Can you work these out from the model? Positions are in its coordinate system, mm. Face numbers are marked on the shaded views. A direction names the side the tool comes from. Round coordinates to 2 decimals unless told otherwise and drop trailing zeros. Order: outer loops, then holes, each group sorted by start corner. A loop starts at its lowest first (then second) coordinate and runs counter-clockwise, first axis right, second up.
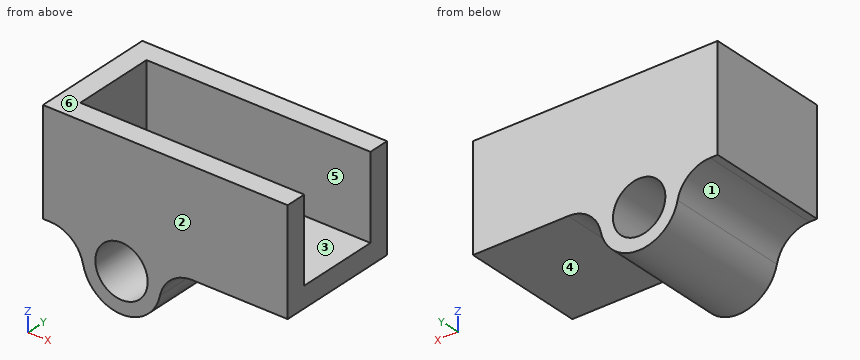
from build123d import *

# Parameters (mm, degrees)
SKETCH1_R           = 2
BOSS_EXTRUDE1_DEPTH = 9.525
FILLET1_R           = 2.54
BOSS_EXTRUDE2_DEPTH = 6.35


with BuildPart() as part:
    # Sketch1 → Boss-Extrude1 (new body)
    with BuildSketch(Plane(origin=(0, 0, 0), x_dir=(1, 0, 0), z_dir=(0, 1, 0))):
        with BuildLine():
            Line((-6, -1.4125), (-6, -3))
            Line((-6, -3), (12.7, -3))
            Line((12.7, -3), (12.7, -1.4125))
            Line((12.7, -1.4125), (2.646666535, -1.4125))
            ThreePointArc((2.646666535, -1.4125), (0, 3), (-2.646666535, -1.4125))
            Line((-2.646666535, -1.4125), (-6, -1.4125))
        make_face()
        Circle(SKETCH1_R, mode=Mode.SUBTRACT)
    extrude(amount=BOSS_EXTRUDE1_DEPTH)

    # Fillet1
    fillet1_edges = [part.edges().sort_by_distance(p)[0] for p in [
        (-2.646666535, 4.7625, 1.4125),
        (2.646666535, 4.7625, 1.4125),
    ]]
    fillet(fillet1_edges, radius=FILLET1_R)

    # Sketch2 → Boss-Extrude2 (add)
    with BuildSketch(Plane.XY.offset(3)):
        Polygon((12.7, 0), (-6, 0), (-6, 9.525), (12.7, 9.525), (12.7, 7.9375), (-4.4125, 7.9375), (-4.4125, 1.5875), (12.7, 1.5875), align=None)
    extrude(amount=BOSS_EXTRUDE2_DEPTH)


solid = part.part
(1) On a 3-axis mill with a long thin cutter (end or side, diameter ignored), from which of +Z, -Z, +X, -X, +Y, -Y can I reach the whole of each face in a straight line? I mean the marked faces 4, 5 and 6. Say none if no direction works.
(2) Please list where these lines run through material, in increasing order: probe 1 along Y at (x, z) = (1.5, 7.75) (1 decimal); probe 2 along X at (y, z) = (6, 7); probe 3 along X at (y, z) = (4.75, 0).
(3) I want a section at B-B, the plane z = 0. List the corners of the cut face in (x, y) for me (3 decimals).
(4) If we mould it in two halves opening along Y, with no side actions, what happens to the marked faces 1, 2 and 3? For each: pulls with the +Y half, pulls with the -Y half, needs draft (parallel to the pull), parting line crosses it, or undercut.
(5) I'm going to push flat-ended pins straight in: pin 1 Ø2 at (x, y) = (7.5, 6.5) entering from -Z; pin 2 Ø3 at (y, z) = (4.5, 7.5) entering from +X; pin 3 Ø3 at (x, y) = (1, 4.5) entering from +Z; pin 4 Ø2 at (x, z) = (5, -0.5) entering from +Y. Where does each tip first touch, or does it pass through?
(6) I want a section at A-A, the plane y = 7.5. List the corners of the cut face in (x, z) for me.
(7) I want a section at D-D, the plane z = 7. List the corners of the cut face in (x, y) for me (1 decimal).
Ans:
1. face 4: -Z, +X, +Y, -Y
1. face 5: +Z, +X
1. face 6: +Z, +X, -X, +Y, -Y
2. probe 1: y = 0 to 1.6, 7.9 to 9.5
2. probe 2: x = -6 to -4.41
2. probe 3: x = -3.15 to -2, 2 to 3.15
3. outline: (-3.148, 0) - (-2, 0) - (-2, 9.525) - (-3.148, 9.525) - close; (2, 0) - (3.148, 0) - (3.148, 9.525) - (2, 9.525) - close
4. face 1: needs draft
4. face 2: pulls with the -Y half
4. face 3: undercut
5. pin 1: stops at z = 1.41
5. pin 2: stops at x = -4.41
5. pin 3: stops at z = 3
5. pin 4: passes through
6. outline: (-6, 1.41) - (-5.42, 1.41) arc R2.54 cw to (-2.94, -0.61) arc R3 ccw to (2.94, -0.61) arc R2.54 cw to (5.42, 1.41) - (12.7, 1.41) - (12.7, 3) - (-4.41, 3) - (-4.41, 9.35) - (-6, 9.35) - close; hole circle Ø4 at (0, 0)
7. outline: (-6, 0) - (12.7, 0) - (12.7, 1.6) - (-4.4, 1.6) - (-4.4, 7.9) - (12.7, 7.9) - (12.7, 9.5) - (-6, 9.5) - close
